The listing builds one solid part. Answer for the finished solid, in the listing's coordinates (mm). Face numbers are marked on the shaded views. A direction names the side the tool comes from. Give positions to 0.01 mm unless a question says otherwise; leave off trailing zeros. Order: outer loops, then holes, each group sorted by start corner. A loop starts at its lowest first (then second) coordinate and runs counter-clockwise, first axis right, second up. Notation, with made-up numbers: (51.5, -21.5) -> (105.5, -21.5) arc R38 ccw to (105.5, 17.5) -> close; hole circle Ø2 at (55, -3). An arc over 180 degrees is marked (long way). One line per question, with ' | ' between items. Start each with the question number.
Autodesk Inventor part; units mm, degrees
ref_plane "YZ Plane" through (0, 0, 0) normal (1, 0, 0) x (0, 1, 0)
ref_plane "XZ Plane" through (0, 0, 0) normal (0, 1, 0) x (-1, 0, 0)
ref_plane "XY Plane" through (0, 0, 0) normal (0, 0, 1) x (1, 0, 0)
sketch "Sketch1" plane through (0, 0, 0) normal (0, 1, 0) x (-1, 0, 0)
  circle A0 centre (0, 0) radius 15
  line L0 (14.942, 1.3178) -> (11.506, 0)
  line L1 (11.506, 0) -> (14.942, -1.3178)
  line L2 (14.3415, 4.3956) -> (11.2545, 2.3922)
  line L3 (11.2545, 2.3922) -> (14.8895, 1.8176)
  line L4 (13.1142, 7.2813) -> (10.5112, 4.6799)
  line L5 (10.5112, 4.6799) -> (14.1862, 4.8736)
  line L6 (11.3137, 9.8488) -> (9.3085, 6.763)
  line L7 (9.3085, 6.763) -> (12.8629, 7.7166)
  line L8 (9.0188, 11.9859) -> (7.699, 8.5506)
  line L9 (7.699, 8.5506) -> (10.9775, 10.2223)
  line L10 (6.3297, 13.5991) -> (5.753, 9.9645)
  line L11 (5.753, 9.9645) -> (8.6123, 12.2812)
  line L12 (3.364, 14.6179) -> (3.5555, 10.9428)
  line L13 (3.5555, 10.9428) -> (5.8706, 13.8035)
  line L14 (0.2513, 14.9979) -> (1.2027, 11.4429)
  line L15 (1.2027, 11.4429) -> (2.8725, 14.7224)
  line L16 (-2.8725, 14.7224) -> (-1.2027, 11.4429)
  line L17 (-1.2027, 11.4429) -> (-0.2513, 14.9979)
  line L18 (-5.8706, 13.8035) -> (-3.5555, 10.9428)
  line L19 (-3.5555, 10.9428) -> (-3.364, 14.6179)
  line L20 (-8.6123, 12.2812) -> (-5.753, 9.9645)
  line L21 (-5.753, 9.9645) -> (-6.3297, 13.5991)
  line L22 (-10.9775, 10.2223) -> (-7.699, 8.5506)
  line L23 (-7.699, 8.5506) -> (-9.0188, 11.9859)
  line L24 (-12.8629, 7.7166) -> (-9.3085, 6.763)
  line L25 (-9.3085, 6.763) -> (-11.3137, 9.8488)
  line L26 (-14.1862, 4.8736) -> (-10.5112, 4.6799)
  line L27 (-10.5112, 4.6799) -> (-13.1142, 7.2813)
  line L28 (-14.8895, 1.8176) -> (-11.2545, 2.3922)
  line L29 (-11.2545, 2.3922) -> (-14.3415, 4.3956)
  line L30 (-14.942, -1.3178) -> (-11.506, 0)
  line L31 (-11.506, 0) -> (-14.942, 1.3178)
  line L32 (-14.3415, -4.3956) -> (-11.2545, -2.3922)
  line L33 (-11.2545, -2.3922) -> (-14.8895, -1.8176)
  line L34 (-13.1142, -7.2813) -> (-10.5112, -4.6799)
  line L35 (-10.5112, -4.6799) -> (-14.1862, -4.8736)
  line L36 (-11.3137, -9.8488) -> (-9.3085, -6.763)
  line L37 (-9.3085, -6.763) -> (-12.8629, -7.7166)
  line L38 (-9.0188, -11.9859) -> (-7.699, -8.5506)
  line L39 (-7.699, -8.5506) -> (-10.9775, -10.2223)
  line L40 (-6.3297, -13.5991) -> (-5.753, -9.9645)
  line L41 (-5.753, -9.9645) -> (-8.6123, -12.2812)
  line L42 (-3.364, -14.6179) -> (-3.5555, -10.9428)
  line L43 (-3.5555, -10.9428) -> (-5.8706, -13.8035)
  line L44 (-0.2513, -14.9979) -> (-1.2027, -11.4429)
  line L45 (-1.2027, -11.4429) -> (-2.8725, -14.7224)
  line L46 (2.8725, -14.7224) -> (1.2027, -11.4429)
  line L47 (1.2027, -11.4429) -> (0.2513, -14.9979)
  line L48 (5.8706, -13.8035) -> (3.5555, -10.9428)
  line L49 (3.5555, -10.9428) -> (3.364, -14.6179)
  line L50 (8.6123, -12.2812) -> (5.753, -9.9645)
  line L51 (5.753, -9.9645) -> (6.3297, -13.5991)
  line L52 (10.9775, -10.2223) -> (7.699, -8.5506)
  line L53 (7.699, -8.5506) -> (9.0188, -11.9859)
  line L54 (12.8629, -7.7166) -> (9.3085, -6.763)
  line L55 (9.3085, -6.763) -> (11.3137, -9.8488)
  line L56 (14.1862, -4.8736) -> (10.5112, -4.6799)
  line L57 (10.5112, -4.6799) -> (13.1142, -7.2813)
  line L58 (14.8895, -1.8176) -> (11.2545, -2.3922)
  line L59 (11.2545, -2.3922) -> (14.3415, -4.3956)
  dimension "d0" = 30
  dimension "d3" = 360
extrude "Extrusion1" add sketch "Sketch1" along normal blind 5 contours L0 L1 A0 L58 L59 L56 L57 L54 L55 L52 L53 L50 L51 L48 L49 L46 L47 L44 L45 L42 L43 L40 L41 L38 L39 L36 L37 L34 L35 L32 L33 L30 L31 L28 L29 L26 L27 L24 L25 L22 L23 L20 L21 L18 L19 L16 L17 L14 L15 L12 L13 L10 L11 L8 L9 L6 L7 L4 L5 L2 L3
sketch "Sketch2" plane through (0, 0, 0) normal (0, -1, 0) x (1, 0, 0)
  circle A0 centre (0, 0) radius 10.5
  circle A1 centre (0, 0) radius 7.5
  dimension "d7" = 3
  dimension "d8" = 15
extrude "Extrusion2" cut sketch "Sketch2" against normal blind 3
sketch "Sketch3" plane through (0, 5, 0) normal (0, 1, 0) x (1, 0, 0)
  circle A0 centre (0, 0) radius 10
  dimension "d11" = 20
extrude "Extrusion3" add sketch "Sketch3" along normal blind 10
properties part number "PlanetaryGear"
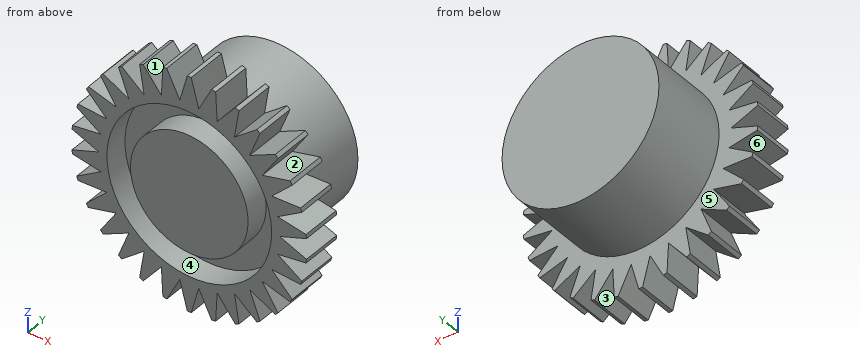
(1) Consider line 1 (Z direction, x = 0, y = 1.5); line 2 (X direction, y = 2, z = -3.25); line 3 (X direction, y = 13, z = 0.25). Determine where each line is inside the solid, lowest interval first.
(2) Given P1, Ø5, axis at y = 8, z = -8.5, coming from the -X side; P2, Ø1.5, axis at x = 6.5, y = 12, coming from the -Z side; P3, Ø1.5, axis at x = -4, y = 5, coming from the +Z side, each flat-ended and moving along its own axis, determine where each tip first touches the part or whether it passes through.
(3) For the marked faces 1, 2 and 3, determine the directions among +Z, -Z, +X, -X, +Y, -Y from which every point of the face is accessible in a straight line to the end or side of a thin tool.
(4) The part is cut by section C-C on y = 5.5. Determine the outline of the cut face in (x, z), plus the area to 3 significant figures.
(5) Determine the mould class of the marked faces 4, 5 and 6 for opening direction X: pulls with the +X half, pulls with the -X half, needs draft (parallel to the pull), parting line crosses it, or undercut.
(6) The part is cut by section A-A on z = 12.75. Determine the outline of the cut face in (x, y), plus the area to 3 significant figures.
(7) The part is cut by section D-D on z = -3. Determine the outline of the cut face in (x, y), plus the area to 3 significant figures.
(8) The part is cut by section B-B on x = -2.25. Determine the outline of the cut face in (y, z), plus the area to 3 significant figures.
Result sheet:
1) line 1: z = -15 to -10.5, -7.5 to 7.5, 10.5 to 15 | line 2: x = -12.58 to -9.98, -6.76 to 6.76, 9.98 to 12.58 | line 3: x = -10 to 10
2) P1: stops at x = -8 | P2: stops at z = -8.18 | P3: stops at z = 14.64
3) face 1: +Z, +Y, -Y | face 2: +Y, -Y | face 3: -Z, +Y, -Y
4) outline: circle Ø20 at (0, 0) | area: 314 mm^2
5) face 4: undercut | face 5: needs draft | face 6: pulls with the -X half
6) outline: (-6.19, 0) -> (-5.02, 0) -> (-5.02, 5) -> (-6.19, 5) -> close; (-3.46, 0) -> (-1.87, 0) -> (-1.87, 5) -> (-3.46, 5) -> close; (-0.85, 0) -> (0.85, 0) -> (0.85, 5) -> (-0.85, 5) -> close; (1.87, 0) -> (3.46, 0) -> (3.46, 5) -> (1.87, 5) -> close; (5.02, 0) -> (6.19, 0) -> (6.19, 5) -> (5.02, 5) -> close | area: 36.2 mm^2
7) outline: (-12.19, 0) -> (-10.06, 0) -> (-10.06, 3) -> (-6.87, 3) -> (-6.87, 0) -> (6.87, 0) -> (6.87, 3) -> (10.06, 3) -> (10.06, 0) -> (12.19, 0) -> (12.19, 5) -> (9.54, 5) -> (9.54, 15) -> (-9.54, 15) -> (-9.54, 5) -> (-12.19, 5) -> close | area: 294 mm^2
8) outline: (0, -13.5) -> (5, -13.5) -> (5, -9.74) -> (15, -9.74) -> (15, 9.74) -> (5, 9.74) -> (5, 13.5) -> (0, 13.5) -> (0, 10.26) -> (3, 10.26) -> (3, 7.15) -> (0, 7.15) -> (0, -7.15) -> (3, -7.15) -> (3, -10.26) -> (0, -10.26) -> close | area: 311 mm^2
